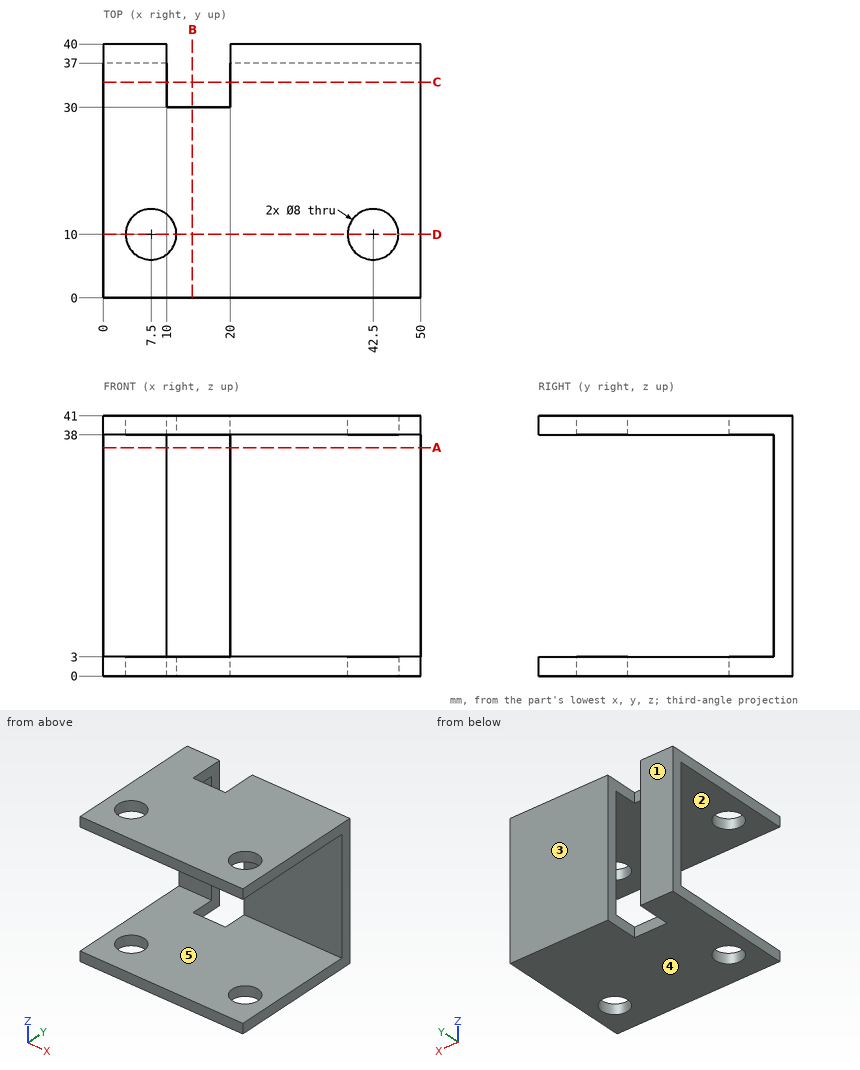
Geometry check sheet. Reference: drawing and pictorial views, mm from the part's lowest x, y, z. A direction names the side the tool comes from. Give positions to 0.01 mm unless a question says otherwise; leave off trailing zeros. Loops run counter-clockwise (first coordinate to the right, second up) from the corner with the lowest first, then second, coordinate; pieces in that order, holes last. Notation, with made-up numbers: (16, 21.25) - (59, 21.25) arc R14 cw to (59, 33.25) - close; hole circle Ø6 at (-3.75, -23.75). An arc over 180 degrees is marked (long way). Use CSV: the item, a comma, the result in double quotes. Start each with the question number.
Q1. Access from +Z, -Z, +X, -X, +Y, -Y to the whole of each face (thin tool, end or side, straight path). Record for the marked faces 1 and 2.
Q2. Section check B-B, the plane x = 14. Record the cut outline in (y, z).
Q3. Go/stop test with flat-tipped pins: pin 1 Ø10.5 at (x, y) = (7.5, 10) entering from +Z; pin 2 Ø12 at (x, z) = (34.5, 27) entering from -Y; pin 3 Ø1.5 at (x, z) = (13.5, 40) entering from +Y; pin 4 Ø7 at (x, y) = (7.5, 10) entering from -Z. Record where each tip stops, or that it passes through.
Q4. Section check D-D, the plane y = 10. Record the cut outline in (x, z), and give its area (3 significant figures).
Q5. Section check A-A, the plane z = 36. Record the cut outline in (x, y), and give its area (3 significant figures).
Q6. Release check for a two-part mould opening along Z. For the marked faces 3, 4 and 5 record: +Z half, -Z half, draft (parallel to the pull), parting line (faces both ways), or undercut.
Q7. Scan lines: probe 1 along Z at (x, y) = (40, 15); probe 2 along Y at (x, z) = (42.5, 39.35); probe 3 along Y at (x, z) = (29.5, 14.5). Record each from-to range of solid material in increasing order. Write a range as from..to.
Q8. Section check C-C, the plane y = 34. Record the cut outline in (x, z), and give its area (3 significant figures).
Findings below:
1,face 1,"+Z, -Z, +X, -X, +Y"
1,face 2,"+X, -X, -Y"
2,outline,"(0, 0) - (30, 0) - (30, 3) - (0, 3) - close; (0, 38) - (30, 38) - (30, 41) - (0, 41) - close"
3,pin 1,"stops at z = 41"
3,pin 2,"stops at y = 37"
3,pin 3,"stops at y = 30"
3,pin 4,"passes through"
4,outline,"(0, 0) - (3.5, 0) - (3.5, 3) - (0, 3) - close; (0, 38) - (3.5, 38) - (3.5, 41) - (0, 41) - close; (11.5, 0) - (38.5, 0) - (38.5, 3) - (11.5, 3) - close; (11.5, 38) - (38.5, 38) - (38.5, 41) - (11.5, 41) - close; (46.5, 0) - (50, 0) - (50, 3) - (46.5, 3) - close; (46.5, 38) - (50, 38) - (50, 41) - (46.5, 41) - close"
4,area,"204 mm^2"
5,outline,"(0, 37) - (10, 37) - (10, 40) - (0, 40) - close; (20, 37) - (50, 37) - (50, 40) - (20, 40) - close"
5,area,"120 mm^2"
6,face 3,"draft"
6,face 4,"-Z half"
6,face 5,"undercut"
7,probe 1,"z = 0..3, 38..41"
7,probe 2,"y = 0..6, 14..40"
7,probe 3,"y = 37..40"
8,outline,"(0, 0) - (10, 0) - (10, 3) - (0, 3) - close; (0, 38) - (10, 38) - (10, 41) - (0, 41) - close; (20, 0) - (50, 0) - (50, 3) - (20, 3) - close; (20, 38) - (50, 38) - (50, 41) - (20, 41) - close"
8,area,"240 mm^2"
